The listing builds one solid part. Answer for the finished solid, in the listing's coordinates (mm). A direction names the side the tool comes from. Round coordinates to 2 decimals unless told otherwise and drop trailing zeros. Order: outer loops, then holes, each group sorted by start corner. A loop starts at its lowest first (then second) coordinate and runs counter-clockwise, first axis right, second up. Notation, with made-up numbers: (56, 14.5) -> (66, 14.5) arc R27 ccw to (66, 50.5) -> close; hole circle Ø5 at (10.5, 31.25). An arc over 180 degrees is marked (long way). Return JSON: item names as keys, results as strings. Group by question number.
(1) The part is cut by section C-C (x = 5.5). Determine the outline of the cut face in (y, z), plus the area to 3 significant figures.
(2) Which of the six approach directions +Z, -Z, +X, -X, +Y, -Y give full straight-line access (tool end or side, diameter ignored) to faces 1 (the face through (9, 8, 3)), 2 (the face through (4, 13, 3))?
(3) The part is cut by section B-B (z = 1.65). Determine the outline of the cut face in (x, y), plus the area to 3 significant figures.
(4) The part is cut by section A-A (y = 13.5). Determine the outline of the cut face in (x, z).
(5) Consider line 1 (X direction, y = 13.5, z = 3.3); line 2 (Y direction, x = 3.75, z = 3.7). Determine where each line is inside the solid, lowest interval first. Write a range as [from, to].
(6) This flat-tipped pin is pushed along its axis until it touches: pin 1 (2.5 mm diameter, centred on x = 4.5, z = 3, fed in from +Y). Where does it stop, or does it pass through?
(7) Determine the mould class of faces 3 (the face through (1, 16, 3)), 4 (the face through (3, 14, 3)), 5 (the face through (0, 8, 3)) for opening direction X: +X half, -X half, draft (parallel to the pull), parting line (faces both ways), or undercut.
from build123d import *

# Parameters (mm, degrees)
SKETCH_1_W          = 9
SKETCH_1_H          = 16
EXTRUDE_1_DEPTH     = 5.5
SKETCH_2_W          = 3
SKETCH_2_H          = 3
CUT_EXTRUDE_1_DEPTH = 20.163767897
FILLET_1_R          = 0.5


with BuildPart() as part:
    # ｽｹｯﾁ1 → ﾎﾞｽ - 押し出し1 (new body)
    with BuildSketch(Plane.XY):
        with Locations((4.5, 8)):
            Rectangle(SKETCH_1_W, SKETCH_1_H)
    extrude(amount=EXTRUDE_1_DEPTH)

    # ｽｹｯﾁ2 → ｶｯﾄ - 押し出し1 (cut, through all)
    with BuildSketch(Plane.XY.offset(5.5)):
        with Locations((4.5, 14.5)):
            Rectangle(SKETCH_2_W, SKETCH_2_H)
    extrude(amount=-CUT_EXTRUDE_1_DEPTH, mode=Mode.SUBTRACT)

    # ﾌｨﾚｯﾄ1
    fillet_1_edges = [part.edges().sort_by_distance(p)[0] for p in [
        (3, 16, 2.75),
        (6, 16, 2.75),
        (0, 16, 2.75),
        (9, 16, 2.75),
    ]]
    fillet(fillet_1_edges, radius=FILLET_1_R)


solid = part.part
Answer below:
{
 "1": {"outline": "(0, 0) -> (13, 0) -> (13, 5.5) -> (0, 5.5) -> close", "area": "71.5 mm²"},
 "2": {"face 1": "+Z, -Z, +X, +Y, -Y", "face 2": "+Z, -Z, +Y"},
 "3": {"outline": "(0, 0) -> (9, 0) -> (9, 15.5) arc R0.5 ccw to (8.5, 16) -> (6.5, 16) arc R0.5 ccw to (6, 15.5) -> (6, 13) -> (3, 13) -> (3, 15.5) arc R0.5 ccw to (2.5, 16) -> (0.5, 16) arc R0.5 ccw to (0, 15.5) -> close", "area": "135 mm²"},
 "4": {"outline": "(0, 0) -> (3, 0) -> (3, 5.5) -> (0, 5.5) -> close; (6, 0) -> (9, 0) -> (9, 5.5) -> (6, 5.5) -> close"},
 "5": {"line 1": "x = [0, 3], [6, 9]", "line 2": "y = [0, 13]"},
 "6": {"pin 1": "stops at y = 13"},
 "7": {"face 3": "draft", "face 4": "undercut", "face 5": "-X half"}
}
